from build123d import *

# Parameters (mm, degrees)
F0_W     = 5
F0_H     = 40
F1_DEPTH = 2.5


with BuildPart() as f1:
    # F0 (on Top) → F1 (new body, symmetric)
    with BuildSketch(Plane.XY):
        with BuildLine():
            Line((-2.5, -21), (2.5, -21))
            ThreePointArc((2.5, -21), (3.207107, -20.707107), (3.5, -20))
            Line((3.5, -20), (3.5, 20))
            ThreePointArc((3.5, 20), (3.207107, 20.707107), (2.5, 21))
            Line((2.5, 21), (-2.5, 21))
            ThreePointArc((-2.5, 21), (-3.207107, 20.707107), (-3.5, 20))
            Line((-3.5, 20), (-3.5, -20))
            ThreePointArc((-3.5, -20), (-3.207107, -20.707107), (-2.5, -21))
        make_face()
        Rectangle(F0_W, F0_H, mode=Mode.SUBTRACT)
    extrude(amount=F1_DEPTH, both=True)


solid = f1.part
Can you work these out from the model? Positions are in its coordinate system, mm. A direction names the side the tool comes from. Give positions to 0.01 mm unless a question says otherwise; leave off trailing zeros. Order: outer loops, then holes, each group sorted by start corner. A loop starts at its lowest first (then second) coordinate and runs counter-clockwise, first axis right, second up. Notation, with made-up numbers: M 15.25,64.5 L 62.25,64.5 A10 ccw 62.25,79.5 Z; hole C 65.25,61.5 d3. An arc over 180 degrees is marked long. One line per item, written item: value.
Item 1: If we section it at C-C on z = -0.8: Write out the boundary of the cut face in (x, y).
Verdict:
outline: M -3.5,-20 A1 ccw -2.5,-21 L 2.5,-21 A1 ccw 3.5,-20 L 3.5,20 A1 ccw 2.5,21 L -2.5,21 A1 ccw -3.5,20 Z; hole M -2.5,-20 L 2.5,-20 L 2.5,20 L -2.5,20 Z
Item 2: For faces 1 (the face through (2.5, 0, 0)), 2 (the face through (0, -21, 0)), which set-ups out of +Z, -Z, +X, -X, +Y, -Y let a thin tool reach every point of the face, with its end or its side?
Verdict:
face 1: +Z, -Z
face 2: +Z, -Z, +X, -X, -Y
Item 3: If we section it at A-A on x = -2: Write out the boundary of the cut face in (y, z).
Verdict:
outline: M -21,-2.5 L -20,-2.5 L -20,2.5 L -21,2.5 Z; M 20,-2.5 L 21,-2.5 L 21,2.5 L 20,2.5 Z
Item 4: If we section it at B-B on y = -7: Write out the boundary of the cut face in (x, z).
Verdict:
outline: M -3.5,-2.5 L -2.5,-2.5 L -2.5,2.5 L -3.5,2.5 Z; M 2.5,-2.5 L 3.5,-2.5 L 3.5,2.5 L 2.5,2.5 Z
Item 5: If we mould it in two halves opening along X, with no side actions, what happens to faces 3 (the face through (-3.215, -20.699, 0.035)), 4 (the face through (3.5, 0, 0)), 5 (the face through (-2.5, 0, 0)), 6 (the face through (0, 20, 0))? For each: pulls with the +X half, pulls with the -X half, needs draft (parallel to the pull), parting line crosses it, or undercut.
Verdict:
face 3: pulls with the -X half
face 4: pulls with the +X half
face 5: undercut
face 6: undercut
Item 6: Please list where these lines run through material, in increasing order: line 1 (X direction, y = 18.5, z = 1.35); line 2 (Y direction, x = 1, z = -1.45); line 3 (Y direction, x = -3, z = 1.05).
Verdict:
line 1: -3.5 to -2.5, 2.5 to 3.5
line 2: -21 to -20, 20 to 21
line 3: -20.87 to 20.87
